```python
from build123d import *

# Parameters (mm, degrees)
F0_W        = 216.7427750782
F0_H        = 304.8
F0_R        = 24.9340536108
F0_W_2      = 149.6857404709
F0_H_2      = 37.9712283611
F1_DEPTH    = 50.8
F2_T1_DEPTH = 50.8
F3_R        = 12.7
F4_SIZE     = 5.08
F6_DEPTH    = 101.6
F6_FACE1_W  = 86.0803631253
F6_FACE1_H  = 101.6
F9_DEPTH    = 101.6
F10_R       = 12.7
F11_R       = 14.8705082973
F12_DEPTH   = 25.4


# Not quite as in the source:
# - a fillet or chamfer that OpenCascade refuses, or shapes differently, is made with other operations: its cross-section is extruded or revolved along the edge and cut away or added


with BuildPart() as f1:
    # F0 (on Top) → F1 (new body)
    with BuildSketch(Plane.XY):
        Rectangle(F0_W, F0_H)
        with Locations((-72.7102532983, -114.1952574253)):
            Circle(F0_R, mode=Mode.SUBTRACT)
        with Locations((0, 96.7190787196)):
            Rectangle(F0_W_2, F0_H_2, mode=Mode.SUBTRACT)
    extrude(amount=F1_DEPTH)

    # F2: fillet of radius 19.05 on 4 edges, made by hand

    # F2_s2 → F2_t1 (join)
    with BuildSketch(Plane.XY):
        with BuildLine():
            ThreePointArc((-74.8428702354, 96.6546929002), (-69.263254417, 110.1250770818), (-55.7928702354, 115.7046929002))
            Line((-55.7928702354, 115.7046929002), (-74.8428702354, 115.7046929002))
            Line((-74.8428702354, 115.7046929002), (-74.8428702354, 96.6546929002))
        make_face()
        with BuildLine():
            ThreePointArc((-55.7928702354, 77.7334645391), (-69.263254417, 83.3130803574), (-74.8428702354, 96.7834645391))
            Line((-74.8428702354, 96.7834645391), (-74.8428702354, 77.7334645391))
            Line((-74.8428702354, 77.7334645391), (-55.7928702354, 77.7334645391))
        make_face()
        with BuildLine():
            ThreePointArc((74.8428702354, 96.7834645391), (69.263254417, 83.3130803574), (55.7928702354, 77.7334645391))
            Line((55.7928702354, 77.7334645391), (74.8428702354, 77.7334645391))
            Line((74.8428702354, 77.7334645391), (74.8428702354, 96.7834645391))
        make_face()
        with BuildLine():
            ThreePointArc((74.8428702354, 96.6546929002), (69.263254417, 110.1250770818), (55.7928702354, 115.7046929002))
            Line((55.7928702354, 115.7046929002), (74.8428702354, 115.7046929002))
            Line((74.8428702354, 115.7046929002), (74.8428702354, 96.6546929002))
        make_face()
    extrude(amount=F2_T1_DEPTH)

    # F3
    f3_edges = [f1.edges().sort_by_distance(p)[0] for p in [
        (108.371388, 152.4, 25.4),
        (-108.371388, 152.4, 25.4),
        (-108.371388, -152.4, 25.4),
        (108.371388, -152.4, 25.4),
    ]]
    fillet(f3_edges, radius=F3_R)

    # F4
    f4_edges = [f1.edges().sort_by_distance(p)[0] for p in [
        (0, -152.4, 50.8),
        (108.371388, 0, 50.8),
        (104.651644, -148.680256, 50.8),
        (-108.371388, 0, 50.8),
        (-104.651644, -148.680256, 50.8),
        (-104.651644, 148.680256, 50.8),
        (0, 152.4, 50.8),
        (104.651644, 148.680256, 50.8),
    ]]
    chamfer(f4_edges, length=F4_SIZE)

    # F5 (on face) → F6 (join)
    with BuildSketch(Plane.XY.offset(50.8)):
        Polygon((26.1903759085, -43.1183193231), (-44.0938870282, 7.8987490062), (-88.495139861, -54.1171146365), (-18.5043358385, -104.2281540196), align=None)
    extrude(amount=F6_DEPTH)

    # F7 (on face) + F6_face1 (on face) → F9 (cut)
    with BuildSketch(Plane(origin=(37.6086943592, -27.5063704871, 0), x_dir=(0.590339639, 0.8071549484, 0), z_dir=(0.8071549484, -0.590339639, 0))):
        Polygon((-57.197030481, 50.8), (-37.1219477484, 152.4), (-95.0521132136, 152.4), (-95.0521132136, 50.8), align=None)
        Polygon((-19.3419477484, 50.8), (-19.3419477484, 152.4), (-39.417030481, 50.8), align=None)
    with BuildSketch(Plane(origin=(-53.4997378497, -79.172634328, 101.6), x_dir=(0.8130867655, -0.5821425185, 0), z_dir=(-0.5821425185, -0.8130867655, 0))):
        Rectangle(F6_FACE1_W, F6_FACE1_H)
    extrude(amount=-F9_DEPTH, dir=(0.8071549484, -0.590339639, 0), mode=Mode.SUBTRACT)

    # F10 (call 1 of 2: OpenCascade refuses the feature's edges together)
    f10_edges = [f1.edges().sort_by_distance(p)[0] for p in [
        (20.942257, -50.293927, 152.4),
    ]]
    fillet(f10_edges, radius=F10_R)

    # F10#2 (call 2 of 2)
    f10_2_edges = [f1.edges().sort_by_distance(p)[0] for p in [
        (-49.178316, 0.797255, 152.4),
    ]]
    fillet(f10_2_edges, radius=F10_R)

    # F11 (on face) → F12 (cut)
    with BuildSketch(Plane(origin=(-38.199850732, -52.2295921019, 12.7856660343), x_dir=(0.8152262825, -0.5625326873, 0.1377065143), z_dir=(-0.5791425631, -0.7918454983, 0.1938416841))):
        with Locations((20.26450634, 108.0148071051)):
            Circle(F11_R)
    extrude(amount=-F12_DEPTH, mode=Mode.SUBTRACT)


solid = f1.part
```
The model under review builds one solid part; all positions refer to its coordinate system, in mm. A direction names the side the tool comes from. Round coordinates to 2 decimals unless told otherwise and drop trailing zeros. Loops run counter-clockwise (first coordinate to the right, second up) from the corner with the lowest first, then second, coordinate; pieces in that order, holes last. Notation, with made-up numbers: (-4, 72.25) - (25, 72.25) arc R22 cw to (25, 110.25) - close; hole circle Ø2 at (38.25, 75.25). An arc over 180 degrees is marked (long way). Use a Markdown table: item, result. Add a question column.
Q1. Machinability: for faces 5 (the face through (-1, 152.4, 23)), 6 (the face through (-69.09, 83.14, 25.04)), which of the approach directions +Z, -Z, +X, -X, +Y, -Y give a long, thin tool a straight path to every point of the face, cutting with its end or side? Answer none if there is none.
Q2. Add section A-A (x = 43). State the section outline as (y, z) points, plus the area to 3 significant figures.
Q3. Add section D-D (z = 86). State the section outline as (x, y) points (3 decimals).
Q4. Insertion check: pin 1 Ø2 at (y, z) = (-15.5, 109) entering from -X; pin 2 Ø10 at (x, y) = (50.5, -113.5) entering from +Z. Each pin has a flat end and moves straight along its axis. Give the tip position at first contact, or say it passes through.
Q5. For probe 1 along Y at (x, z) = (38, 16); probe 2 along Y at (x, z) = (-60, 44.5); probe 3 along Y at (x, z) = (-66.5, 24), list the stretches that pass through material, from the lowest coordinate up.
Q6. Add section C-C (z = 31). State the section outline as (x, y) points.
Q7. Add section B-B (y = -129.5). State the section outline as (x, z) points, plus the area to 3 significant figures.
Q8. The part is to be moulded in two halves that separate along Y. For faces 1 (the face through (-24.79, -40.47, 100.89)), 2 (the face through (-25.63, -22.58, 127.08)), 3 (the face through (-1, 115.705, 25)), 4 (the face through (-14.214, -25.853, 102.214)), say which applies: pulls with the +Y half, pulls with the -Y half, needs draft (parallel to the pull), parting line crosses it, or undercut.
Worked answers:
| question | item | result |
|---|---|---|
| 1 | face 5 | +Z, -Z, +X, -X, +Y |
| 1 | face 6 | +Z, -Z |
| 2 | outline | (-152.4, 0) - (77.73, 0) - (77.73, 50.8) - (-147.32, 50.8) - (-152.4, 45.72) - close; (115.7, 0) - (152.4, 0) - (152.4, 45.72) - (147.32, 50.8) - (115.7, 50.8) - close |
| 2 | area | 13,500 mm² |
| 3 | outline | (-61.901, -16.972) - (7.949, -68.059) - (18.445, -53.708) - (-51.55, -2.515) - close |
| 4 | pin 1 | x = -57.62 |
| 4 | pin 2 | z = 50.8 |
| 5 | probe 1 | -152.4 to 77.73, 115.7 to 152.4 |
| 5 | probe 2 | -152.4 to -135.65, -92.74 to 78.2, 115.23 to 152.4 |
| 5 | probe 3 | -152.4 to -138.34, -90.05 to 81.03, 112.41 to 152.4 |
| 6 | outline | (-108.37, -139.7) arc R12.7 ccw to (-95.67, -152.4) - (95.67, -152.4) arc R12.7 ccw to (108.37, -139.7) - (108.37, 139.7) arc R12.7 ccw to (95.67, 152.4) - (-95.67, 152.4) arc R12.7 ccw to (-108.37, 139.7) - close; hole circle Ø49.87 at (-72.71, -114.2); hole (-74.84, 96.72) arc R19.05 ccw to (-55.79, 77.73) - (55.79, 77.73) arc R19.05 ccw to (74.84, 96.72) arc R19.05 ccw to (55.79, 115.7) - (-55.79, 115.7) arc R19.05 ccw to start |
| 7 | outline | (-108.37, 0) - (-92.39, 0) - (-92.39, 50.8) - (-103.29, 50.8) - (-108.37, 45.72) - close; (-53.03, 0) - (108.37, 0) - (108.37, 45.72) - (103.29, 50.8) - (-53.03, 50.8) - close |
| 7 | area | 8,980 mm² |
| 8 | face 1 | pulls with the -Y half |
| 8 | face 2 | undercut |
| 8 | face 3 | undercut |
| 8 | face 4 | pulls with the +Y half |
